from build123d import *

# Parameters (mm, degrees)
SKETCH_1_R               = 63
SKETCH_1_R_2             = 2.5
EXTRUDE_1_DEPTH          = 1
CUT_EXTRUDE_1_DEPTH      = 1
PATTERN_CIRCULAR_1_COUNT = 3


with BuildPart() as part:
    # Sketch 1 → Extrude 1 (new body)
    with BuildSketch(Plane(origin=(0, 0, 0), x_dir=(0, 0, -1), z_dir=(1, 0, 0))):
        Circle(SKETCH_1_R)
        Circle(SKETCH_1_R_2, mode=Mode.SUBTRACT)
    extrude(amount=EXTRUDE_1_DEPTH)

    # Sketch 2 → Cut-Extrude 1 (cut)
    with BuildSketch(Plane.ZY):
        with BuildLine():
            Line((-3, 5.196152423), (-3, 62.92853089))
            ThreePointArc((-3, 62.92853089), (-54.559600438, 31.5), (-55.997706374, -28.866189234))
            Line((-55.997706374, -28.866189234), (-6, 0))
            ThreePointArc((-6, 0), (-5.196152423, 3), (-3, 5.196152423))
        make_face()
    cut_extrude_1 = extrude(amount=-CUT_EXTRUDE_1_DEPTH, mode=Mode.SUBTRACT)

    # Pattern Circular 1: Cut-Extrude 1 ×3 about axis
    pattern_circular_1_axis = Axis((0, 0, 0), (1, 0, 0))
    for i in range(1, PATTERN_CIRCULAR_1_COUNT):
        add(cut_extrude_1.rotate(pattern_circular_1_axis, i * 360 / PATTERN_CIRCULAR_1_COUNT), mode=Mode.SUBTRACT)


solid = part.part
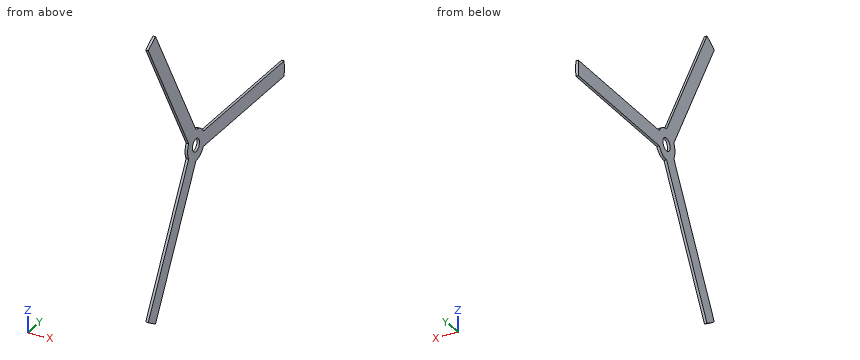
Here's how the part is built. I have some questions about the finished solid (model axes, mm). Round coordinates to 2 decimals unless told otherwise and drop trailing zeros. Loops run counter-clockwise (first coordinate to the right, second up) from the corner with the lowest first, then second, coordinate; pieces in that order, holes last. Notation, with made-up numbers: (-25, -9) - (10, -9) arc R21 cw to (10, 28) - close; hole circle Ø6 at (-35, -35). An arc over 180 degrees is marked (long way). One line per question, with ' | ' between items. Start each with the question number.
Q1. I want a section at C-C (y = 51.5). Write out the boundary of the cut face in (x, z), then the cut area to 3 significant figures.
Q2. I want a section at A-A (z = 0). Write out the boundary of the cut face in (x, y).
Q3. I want a section at D-D (z = 48). Write out the boundary of the cut face in (x, y), then the cut area to 3 significant figures.
Q4. I want a section at B-B (x = 0.2). Write out the boundary of the cut face in (y, z).
Q5. Please list where these lines run through material, in increasing order: line 1 (Y direction, x = 0.7, z = 0); line 2 (Z direction, x = 0.55, y = 25); line 3 (Y direction, x = 0.5, z = -46). Write a range as [from, to].
Response values:
1) outline: (0, -3) - (1, -3) - (1, 3) - (0, 3) - close | area: 6.00 mm²
2) outline: (0, -6) - (1, -6) - (1, -2.5) - (0, -2.5) - close; (0, 2.5) - (1, 2.5) - (1, 63) - (0, 63) - close
3) outline: (0, -31.18) - (1, -31.18) - (1, -24.25) - (0, -24.25) - close | area: 6.93 mm²
4) outline: (-34.06, -53) arc R63 ccw to (-28.87, -56) - (0, -6) arc R6 ccw to (5.2, -3) - (62.93, -3) arc R63 ccw to (62.93, 3) - (5.2, 3) arc R6 ccw to (0, 6) - (-28.87, 56) arc R63 ccw to (-34.06, 53) - (-5.2, 3) arc R6 ccw to (-5.2, -3) - close; hole circle Ø5 at (0, 0)
5) line 1: y = [-6, -2.5], [2.5, 63] | line 2: z = [-3, 3] | line 3: y = [-30.02, -23.09]
